from build123d import *

# Parameters (mm, degrees)
BOSS_EXTRUDE1_DEPTH       = 3
SKETCH2_R                 = 3.6
CUT_EXTRUDE1_DEPTH        = 3.95
BOSS_EXTRUDE2_DEPTH       = 1.64
SKETCH4_R                 = 3.25
CUT_EXTRUDE2_DEPTH        = 4.64
CUT_EXTRUDE3_REACH        = 64.566
SKETCH7_W                 = 12.2
SKETCH7_H                 = 14
BODY_MOVE_COPY1_OUTLINE_R = 3.6
BODY_MOVE_COPY1_DEPTH     = 4.64
BODY_MOVE_COPY1_START     = 3
BODY_MOVE_COPY1_2_DEPTH   = 1.64
BODY_MOVE_COPY1_3_DEPTH   = 4.64
BODY_MOVE_COPY1_4_DEPTH   = 3


# Read off the part's stored shape, not the designer's step: Body-Move/Copy1
with BuildPart() as part:
    # Sketch1 → Boss-Extrude1 (new body)
    with BuildSketch(Plane(origin=(0, 0, 0), x_dir=(1, 0, 0), z_dir=(0, 1, 0))):
        with BuildLine():
            Line((0, 7), (55, 7))
            ThreePointArc((55, 7), (62, 0), (55, -7))
            Line((55, -7), (0, -7))
            ThreePointArc((0, -7), (-7, 0), (0, 7))
        make_face()
    extrude(amount=BOSS_EXTRUDE1_DEPTH)

    # Sketch2 → Cut-Extrude1 (cut)
    with BuildSketch(Plane.XZ):
        with Locations(Location((0, 0, 0), (0, 0, 270))):
            Circle(SKETCH2_R)
    extrude(amount=-CUT_EXTRUDE1_DEPTH, mode=Mode.SUBTRACT)

    # Sketch3 → Boss-Extrude2 (add)
    with BuildSketch(Plane(origin=(0, 3, 0), x_dir=(1, 0, 0), z_dir=(0, 1, 0))):
        with BuildLine():
            Line((0, -7), (55, -7))
            ThreePointArc((55, -7), (62, 0), (55, 7))
            Line((55, 7), (0, 7))
            ThreePointArc((0, 7), (-7, 0), (0, -7))
        make_face()
        with BuildLine():
            Line((14.555396889, 2.01999279), (2.561818442, 2.765860855))
            ThreePointArc((2.561818442, 2.765860855), (-3.77, 0), (2.561818442, -2.765860855))
            Line((2.561818442, -2.765860855), (14.555396889, -2.01999279))
            ThreePointArc((14.555396889, -2.01999279), (16.57, 0), (14.555396889, 2.01999279))
        make_face(mode=Mode.SUBTRACT)
    extrude(amount=BOSS_EXTRUDE2_DEPTH)

    # Sketch4 → Cut-Extrude2 (cut)
    with BuildSketch(Plane(origin=(0, 4.64, 0), x_dir=(1, 0, 0), z_dir=(0, 1, 0))):
        with Locations(Location((55, 0, 0), (0, 0, 270))):
            Circle(SKETCH4_R)
    extrude(amount=-CUT_EXTRUDE2_DEPTH, mode=Mode.SUBTRACT)

    # Sketch7 → Cut-Extrude3 (cut, up to next)
    with BuildSketch(Plane(origin=(0, 4.64, 0), x_dir=(1, 0, 0), z_dir=(0, 1, 0)), mode=Mode.PRIVATE) as cut_extrude3_sk1:
        with Locations((33.6, 0)):
            Rectangle(SKETCH7_W, SKETCH7_H)
    cut_extrude3_tool1 = extrude(cut_extrude3_sk1.sketch, amount=-CUT_EXTRUDE3_REACH, mode=Mode.PRIVATE) & part.part
    add(cut_extrude3_tool1.solids().sort_by_distance((33.6, 4.64, 0))[0], mode=Mode.SUBTRACT)


with BuildPart() as cut_extrude3_piece_1:
    # of the separate pieces the step leaves, piece 1, a body of its own (cut_extrude3_pieces)
    add(part.part.solids().sort_by_distance((0, 0, -7))[0])

    # Body-Move/Copy1 outline → Body-Move/Copy1 (cut)
    # profile 1 of 2: a face of its own
    with BuildSketch(Plane(origin=(0, 0, 0), x_dir=(1, 0, 0), z_dir=(0, 1, 0))):
        with BuildLine():
            Line((0, -7), (12.2, -7))
            ThreePointArc((12.2, -7), (5.2, 0), (12.2, 7))
            Line((12.2, 7), (0, 7))
            ThreePointArc((0, 7), (-7, 0), (0, -7))
        make_face()
        Circle(BODY_MOVE_COPY1_OUTLINE_R, mode=Mode.SUBTRACT)
    # profile 2 of 2: a face of its own
    with BuildSketch(Plane(origin=(0, 0, 0), x_dir=(1, 0, 0), z_dir=(0, 1, 0))):
        with Locations((12.2, 0)):
            Circle(BODY_MOVE_COPY1_OUTLINE_R)
    extrude(amount=BODY_MOVE_COPY1_DEPTH, mode=Mode.SUBTRACT)

    # Body-Move_Copy1 2 outline → Body-Move_Copy1 2 (cut)
    with BuildSketch(Plane(origin=(0, 0, 0), x_dir=(1, 0, 0), z_dir=(0, 1, 0)).offset(BODY_MOVE_COPY1_START)):
        with BuildLine():
            ThreePointArc((26.755396889, -2.01999279), (27.134536032, -1.983061279), (27.5, -1.875606568))
            Line((27.5, -1.875606568), (27.5, 1.875606568))
            ThreePointArc((27.5, 1.875606568), (27.134536032, 1.983061279), (26.755396889, 2.01999279))
            Line((26.755396889, 2.01999279), (14.761818442, 2.765860855))
            ThreePointArc((14.761818442, 2.765860855), (11.91613853, 3.759298161), (9.251901395, 2.349811613))
            Line((9.251901395, 2.349811613), (9.461484137, 2.336777882))
            ThreePointArc((9.461484137, 2.336777882), (12.476666707, 3.58935308), (15.264276596, 1.889499654))
            ThreePointArc((15.264276596, 1.889499654), (16.57, 0), (15.264276596, -1.889499654))
            ThreePointArc((15.264276596, -1.889499654), (12.476666707, -3.58935308), (9.461484137, -2.336777882))
            Line((9.461484137, -2.336777882), (9.251901395, -2.349811613))
            ThreePointArc((9.251901395, -2.349811613), (11.91613853, -3.759298161), (14.761818442, -2.765860855))
            Line((14.761818442, -2.765860855), (26.755396889, -2.01999279))
        make_face()
    extrude(amount=BODY_MOVE_COPY1_2_DEPTH, mode=Mode.SUBTRACT)

    # Body-Move_Copy1 3 outline → Body-Move_Copy1 3 (add)
    with BuildSketch(Plane(origin=(0, 0, 0), x_dir=(1, 0, 0), z_dir=(0, 1, 0))):
        with BuildLine():
            Line((27.5, -7), (39.7, -7))
            Line((39.7, -7), (39.7, 7))
            Line((39.7, 7), (27.5, 7))
            Line((27.5, 7), (27.5, 1.875606568))
            ThreePointArc((27.5, 1.875606568), (28.77, 0), (27.5, -1.875606568))
            Line((27.5, -1.875606568), (27.5, -7))
        make_face()
        with BuildLine():
            ThreePointArc((5.689385292, 2.571360753), (5.2, 0), (5.689385292, -2.571360753))
            Line((5.689385292, -2.571360753), (9.251901395, -2.349811613))
            ThreePointArc((9.251901395, -2.349811613), (8.43, 0), (9.251901395, 2.349811613))
            Line((9.251901395, 2.349811613), (5.689385292, 2.571360753))
        make_face()
    extrude(amount=BODY_MOVE_COPY1_3_DEPTH)

    # Body-Move_Copy1 4 outline → Body-Move_Copy1 4 (add)
    with BuildSketch(Plane(origin=(0, 0, 0), x_dir=(1, 0, 0), z_dir=(0, 1, 0))):
        with BuildLine():
            Line((27.5, 1.875606568), (27.5, -1.875606568))
            ThreePointArc((27.5, -1.875606568), (28.77, 0), (27.5, 1.875606568))
        make_face()
    extrude(amount=BODY_MOVE_COPY1_4_DEPTH)


with BuildPart() as cut_extrude3_piece_2:
    # of the separate pieces the step leaves, piece 2, a body of its own (cut_extrude3_pieces)
    add(part.part.solids().sort_by_distance((39.7, 0, -7))[0])


with BuildPart() as cut_extrude3_piece_1_1:
    add(cut_extrude3_piece_1.part)

    # Combine1: union Cut-Extrude3 piece 2
    add(cut_extrude3_piece_2.part)


solid = cut_extrude3_piece_1_1.part
The model under review builds one solid part; all positions refer to its coordinate system, in mm. A direction names the side the tool comes from. Round coordinates to 2 decimals unless told otherwise and drop trailing zeros. Order: outer loops, then holes, each group sorted by start corner. A loop starts at its lowest first (then second) coordinate and runs counter-clockwise, first axis right, second up. Notation, with made-up numbers: (4.5, 21) -> (53.5, 21) arc R20 ccw to (53.5, 48) -> close; hole circle Ø11 at (4.25, 89). An arc over 180 degrees is marked (long way). Return JSON: item names as keys, results as strings.
1. Take a section at D-D (x = 10). Write out the cut boundary in (y, z).
Answer block:
{"outline": "(0, -6.65) -> (4.64, -6.65) -> (4.64, -3.06) -> (3, -3.06) -> (3, -2.85) -> (0, -2.85) -> close; (0, 2.85) -> (3, 2.85) -> (3, 3.06) -> (4.64, 3.06) -> (4.64, 6.65) -> (0, 6.65) -> close"}
2. For faces 4 (the face through (62, 2, 0)), 5 (the face through (20.67, 3.81, 2.4)), list the 3-axis set-ups (+Z, -Z, +X, -X, +Y, -Y) from which the entire face can be reached by the end or side of a thin tool; tool diameter is ignored.
Answer block:
{"face 4": "+X, +Y, -Y", "face 5": "+Y"}
3. For L1, parallel to Z at x = 12.2, y = 1.2; L2, parallel to X at y = 1.45, z = -2.25; L3, parallel to X at y = 2.8, z = -2.75, list the stretches that pass through material, from the lowest coordinate up. Write a range as [from, to].
Answer block:
{"L1": "z = [-7, -3.6], [3.6, 7]", "L2": "x = [5.57, 9.39], [15.01, 52.65], [57.35, 61.63]", "L3": "x = [5.76, 9.88], [14.52, 53.27], [56.73, 61.44]"}
4. Take a section at B-B (x = 57.5). Write out the cut boundary in (y, z), then the cut area to 3 significant figures.
Answer block:
{"outline": "(0, -6.54) -> (4.64, -6.54) -> (4.64, -2.08) -> (0, -2.08) -> close; (0, 2.08) -> (4.64, 2.08) -> (4.64, 6.54) -> (0, 6.54) -> close", "area": "41.4 mm²"}
5. Insertion check: P1, Ø4, axis at x = 55, z = 0, coming from the -Y side. The pin has a flat end and moves straight along its axis. Give the tip position at first contact, or say it passes through.
Answer block:
{"P1": "passes through"}
6. The part is to be moulded in two halves that separate along Z. For faces 1 (the face through (5.2, 2.29, 0.15)), 2 (the face through (33, 4.64, 0)), 3 (the face through (51.827, 2.352, -0.705)), say which applies: +Z half, -Z half, draft (parallel to the pull), parting line (faces both ways), or undercut.
Answer block:
{"face 1": "parting line", "face 2": "draft", "face 3": "undercut"}
7. Take a section at C-C (y = 4). Write out the cut boundary in (x, z).
Answer block:
{"outline": "(12.2, -7) -> (55, -7) arc R7 ccw to (55, 7) -> (12.2, 7) arc R7 ccw to start; hole (14.76, -2.77) -> (26.76, -2.02) arc R2.02 ccw to (26.76, 2.02) -> (14.76, 2.77) arc R3.77 ccw (long way) to start; hole circle Ø6.5 at (55, 0)"}
8. Take a section at A-A (z = 0). Write out the cut boundary in (x, y).
Answer block:
{"outline": "(5.2, 0) -> (8.6, 0) -> (8.6, 3) -> (8.43, 3) -> (8.43, 4.64) -> (5.2, 4.64) -> close; (15.8, 0) -> (51.75, 0) -> (51.75, 4.64) -> (28.77, 4.64) -> (28.77, 3) -> (15.8, 3) -> close; (58.25, 0) -> (62, 0) -> (62, 4.64) -> (58.25, 4.64) -> close"}
